Work out the finished part from the listing and answer in its coordinate system (mm). Round coordinates to 2 decimals unless told otherwise and drop trailing zeros. Order: outer loops, then holes, each group sorted by start corner. A loop starts at its lowest first (then second) coordinate and runs counter-clockwise, first axis right, second up. Notation, with made-up numbers: M -23,2 L -3,2 A22 cw -3,34 Z; hole C 51,47.25 d10. An arc over 180 degrees is marked long. Return JSON: item names as keys, results as strings.
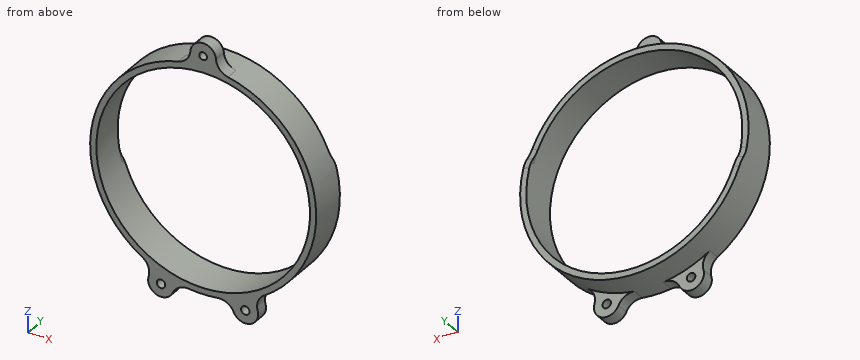
from build123d import *

# Parameters (mm, degrees)
SKETCH_1_R          = 44
SKETCH_1_R_2        = 41.6
EXTRUDE_1_DEPTH     = 15
SKETCH_2_R          = 5
SKETCH_2_R_2        = 1.5
SKETCH_2_R_3        = 1.65
EXTRUDE_2_DEPTH     = 5
FILLET_1_R          = 6
CUT_EXTRUDE_START   = -1.5
CUT_EXTRUDE_1_DEPTH = 1.5
FILLET_2_R          = 10
FILLET_START        = -45
FILLET_3_DEPTH      = 90


with BuildPart() as part:
    # 草图1 → 凸台-拉伸1 (new body)
    with BuildSketch(Plane(origin=(0, 0, 0), x_dir=(1, 0, 0), z_dir=(0, 1, 0))):
        with Locations(Location((0, 0, 0), (0, 0, 270))):
            Circle(SKETCH_1_R)
        with Locations(Location((0, 0, 0), (0, 0, 270))):
            Circle(SKETCH_1_R_2, mode=Mode.SUBTRACT)
    extrude(amount=EXTRUDE_1_DEPTH)

    # 草图2 → 凸台-拉伸2 (add)
    # profile 1 of 3: a face of its own
    with BuildSketch(Plane.XZ):
        with Locations((0, 48)):
            Circle(SKETCH_2_R)
        with Locations(Location((0, 48, 0), (0, 0, 270))):
            Circle(SKETCH_2_R_2, mode=Mode.SUBTRACT)
    # profile 2 of 3: a face of its own
    with BuildSketch(Plane.XZ):
        with Locations((-16.41696688, -45.105245798)):
            Circle(SKETCH_2_R)
        with Locations(Location((-16.41696688, -45.105245798, 0), (0, 0, 270))):
            Circle(SKETCH_2_R_3, mode=Mode.SUBTRACT)
    # profile 3 of 3: a face of its own
    with BuildSketch(Plane.XZ):
        with Locations((16.41696688, -45.105245798)):
            Circle(SKETCH_2_R)
        with Locations(Location((16.41696688, -45.105245798, 0), (0, 0, 90))):
            Circle(SKETCH_2_R_3, mode=Mode.SUBTRACT)
    extrude(amount=-EXTRUDE_2_DEPTH)

    # 圆角1
    fillet_1_edges = [part.edges().sort_by_distance(p)[0] for p in [
        (2.870750936, 2.5, 43.90625),
        (-2.870750936, 2.5, 43.90625),
        (-17.714445389, 2.5, -40.276524485),
        (-12.319198447, 2.5, -42.240233778),
        (12.319198447, 2.5, -42.240233778),
        (17.714445389, 2.5, -40.276524485),
    ]]
    fillet(fillet_1_edges, radius=FILLET_1_R)

    # 草图3 → 切除-拉伸1 (cut)
    with BuildSketch(Plane(origin=(0, 15, 0), x_dir=(1, 0, 0), z_dir=(0, 1, 0)).offset(CUT_EXTRUDE_START)):
        with BuildLine():
            Line((42.117616116, -12.732101662), (39.8202916, -12.03762339))
            ThreePointArc((39.8202916, -12.03762339), (-12.03762339, -39.8202916), (-39.8202916, 12.03762339))
            Line((-39.8202916, 12.03762339), (-42.117616116, 12.732101662))
            ThreePointArc((-42.117616116, 12.732101662), (-12.732101662, -42.117616116), (42.117616116, -12.732101662))
        make_face()
    extrude(amount=CUT_EXTRUDE_1_DEPTH, mode=Mode.SUBTRACT)

    # 圆角2
    # the kernel refuses this fillet: 10 mm, written as the material it adds along each edge
    with BuildSketch(Plane(origin=(-27.214137615, 13.5, -8.22679911), x_dir=(-0.28936594687336814, 0, 0.9572185480808858), z_dir=(-0.9572185480808859, 0, -0.28936594687336814))) as fillet_2_piece_1_section:
        with BuildLine():
            CenterArc((5.267826876, 10), FILLET_2_R, 238.211669383, 31.788330617)
            Line((0, 1.5), (-0.105356538, 1.33))
            ThreePointArc((-0.105356538, 1.33), (-0.2, 0.75), (-0.2, 0))
            Line((-0.2, 0), (0, -0.2))
            Line((0, -0.2), (5.267826876, -0.2))
            Line((5.267826876, -0.2), (5.267826876, 0))
        make_face()
    fillet_2_piece_1 = extrude(amount=28.739134382, mode=Mode.PRIVATE)
    fillet_2_piece_1 = fillet_2_piece_1 & Plane(origin=(0, 13.5, 0), x_dir=(0, 0, 1), z_dir=(0, -1, 0)) * Cylinder(44, 79, mode=Mode.PRIVATE)
    fillet_2_piece_1 = fillet_2_piece_1 - Plane(origin=(0, 13.5, 0), x_dir=(0, 0, 1), z_dir=(0, -1, 0)) * Cylinder(41.6, 79, mode=Mode.PRIVATE)
    add(fillet_2_piece_1)
    with BuildSketch(Plane(origin=(54.723770101, 13.5, 16.542925943), x_dir=(-0.2893659468733635, 0, 0.9572185480808872), z_dir=(-0.9572185480808872, 0, -0.2893659468733635))) as fillet_2_piece_2_section:
        with BuildLine():
            CenterArc((5.267826876, 10), FILLET_2_R, 238.211669383, 31.788330617)
            Line((0, 1.5), (-0.105356538, 1.33))
            ThreePointArc((-0.105356538, 1.33), (-0.2, 0.75), (-0.2, 0))
            Line((-0.2, 0), (0, -0.2))
            Line((0, -0.2), (5.267826876, -0.2))
            Line((5.267826876, -0.2), (5.267826876, 0))
        make_face()
    fillet_2_piece_2 = extrude(amount=28.739134382, mode=Mode.PRIVATE)
    fillet_2_piece_2 = fillet_2_piece_2 & Plane(origin=(0, 13.5, 0), x_dir=(0, 0, 1), z_dir=(0, -1, 0)) * Cylinder(44, 79, mode=Mode.PRIVATE)
    fillet_2_piece_2 = fillet_2_piece_2 - Plane(origin=(0, 13.5, 0), x_dir=(0, 0, 1), z_dir=(0, -1, 0)) * Cylinder(41.6, 79, mode=Mode.PRIVATE)
    add(fillet_2_piece_2)

    # 圆角3: read off the stored shape, not the designer's step
    # 圆角3 outline → 圆角3 (cut)
    with BuildSketch(Plane(origin=(0, 0, 0), x_dir=(0, 1, 0), z_dir=(0.9572185480808874, 0, 0.2893659468733631)).offset(FILLET_START)):
        with BuildLine():
            ThreePointArc((14.25, 1.468155838), (14.810708435, -0.395023527), (15, -2.3315152))
            Line((15, -2.3315152), (15, 0))
            ThreePointArc((15, 0), (14.594692852, 0.718595666), (14.25, 1.468155838))
        make_face()
    extrude(amount=FILLET_3_DEPTH, mode=Mode.SUBTRACT)


solid = part.part
Item 1: Consider line 1 along Z through (x, y) = (-16.5, 2.5); line 2 along Y through (x, z) = (27.5, 32); line 3 along Z through (x, y) = (-28, 9.5). Determine where each line is inside the solid, lowest interval first. Write a range as [from, to].
Output:
{"line 1": "z = [-50.1, -46.75], [-43.46, -38.19], [38.19, 40.79]", "line 2": "y = [0, 13.5]", "line 3": "z = [-33.94, -30.77], [30.77, 33.94]"}
Item 2: Find section A-A (x = 0). Determine the outline of the cut face in (y, z).
Output:
{"outline": "M 0,-44 L 15,-44 L 15,-41.6 L 0,-41.6 Z; M 0,41.6 L 13.5,41.6 L 13.5,44 L 5,44 L 5,46.5 L 0,46.5 Z; M 0,49.5 L 5,49.5 L 5,53 L 0,53 Z"}
Item 3: Find section B-B (z = 0). Determine the outline of the cut face in (x, y), plus the area to 3 significant figures.
Output:
{"outline": "M -44,0 L -41.6,0 L -41.6,13.5 L -44,13.5 Z; M 41.6,0 L 44,0 L 44,15 L 41.6,15 Z", "area": "68.4 mm^2"}
Item 4: Find section C-C (x = 26.5). Determine the outline of the cut face in (y, z).
Output:
{"outline": "M 0,-35.12 L 15,-35.12 L 15,-32.07 L 0,-32.07 Z; M 0,32.07 L 13.5,32.07 L 13.5,35.12 L 0,35.12 Z"}
Item 5: Find section D-D (y = 6.75). Determine the outline of the cut face in (x, z), plus the area to 3 significant figures.
Output:
{"outline": "C 0,0 d88; hole C 0,0 d83.2", "area": "645 mm^2"}
Item 6: Each of these flat-tipped pins is pushed along its axis until it touches: pin 1 (3 mm diameter, centred on x = -2.5, z = 47.5, fed in from +Y); pin 2 (3 mm diameter, centred on x = 18, y = 6, fed in from +Z); pin 3 (5 mm diameter, centred on x = -11, y = 9.5, fed in from -Z); pin 4 (4 mm diameter, centred on x = 19, z = -40.5, fed in from +Y). Where does it stop, or does it pass through?
Output:
{"pin 1": "stops at y = 5", "pin 2": "stops at z = 40.79", "pin 3": "stops at z = -43.17", "pin 4": "stops at y = 15"}
